Read the model definition and answer for the solid it produces. Units are mm, in the model's axes. Face numbers are marked on the shaded views. A direction names the side the tool comes from. Coordinates: 2 decimals unless noted, no trailing zeros. Write each loop counter-clockwise with the first axis right and the second up, starting at its lowest first coordinate (ties: lowest second). Pieces come first, ordered by that corner, then holes. Notation, with made-up numbers: (32.5, 28.25) -> (64.5, 28.25) arc R13 ccw to (64.5, 53.25) -> close; hole circle Ø4 at (-7.5, -39.75). An arc over 180 degrees is marked (long way). One line per item, written item: value. Start each with the question number.
from build123d import *

# Parameters (mm, degrees)
SKETCH1_W           = 82
SKETCH1_H           = 30
SKETCH1_R           = 2
BOSS_EXTRUDE1_DEPTH = 3
BOSS_EXTRUDE2_DEPTH = 42.5
SKETCH4_R           = 12
SKETCH4_R_2         = 1.65
CUT_EXTRUDE2_DEPTH  = 99.459382488
SKETCH7_W           = 19.5
SKETCH7_H           = 30
CUT_EXTRUDE4_DEPTH  = 98.109474306
SKETCH8_W           = 8
SKETCH8_H           = 5
BOSS_EXTRUDE3_DEPTH = 42.5
SKETCH8_3_R         = 1.755
CUT_EXTRUDE5_DEPTH  = 82.317279836
SKETCH9_W           = 4
SKETCH9_H           = 36
CUT_EXTRUDE6_DEPTH  = 80.26380006
SKETCH10_W          = 46.5
SKETCH10_H          = 46.9
SKETCH10_R          = 4.75
BOSS_EXTRUDE4_DEPTH = 3
BOSS_EXTRUDE4_DRAFT = -33
SKETCH12_W          = 8
SKETCH12_H          = 5
BOSS_EXTRUDE6_DEPTH = 3
CUT_EXTRUDE7_DEPTH  = 3
CUT_EXTRUDE8_DEPTH  = 0.25


with BuildPart() as part:
    # Sketch1 → Boss-Extrude1 (new body)
    with BuildSketch(Plane(origin=(0, 0, 0), x_dir=(1, 0, 0), z_dir=(0, 1, 0))):
        with Locations((41, 15)):
            Rectangle(SKETCH1_W, SKETCH1_H)
        with Locations(Location((78, 23.86, 0), (0, 0, 270))):
            Circle(SKETCH1_R, mode=Mode.SUBTRACT)
        with Locations(Location((78, 5, 0), (0, 0, 270))):
            Circle(SKETCH1_R, mode=Mode.SUBTRACT)
    extrude(amount=BOSS_EXTRUDE1_DEPTH)

    # Sketch2 → Boss-Extrude2 (add)
    with BuildSketch(Plane(origin=(0, 3, 0), x_dir=(1, 0, 0), z_dir=(0, 1, 0))):
        Polygon((52.5, 2.5), (10, 2.5), (10, 30), (8, 30), (8, 0), (54.5, 0), (54.5, 30), (52.5, 30), align=None)
    extrude(amount=BOSS_EXTRUDE2_DEPTH)

    # Sketch4 → Cut-Extrude2 (cut, through all)
    with BuildSketch(Plane.XY):
        with Locations((31.25, 24.25)):
            Circle(SKETCH4_R)
        with Locations((16.25, 9.25)):
            Circle(SKETCH4_R_2)
        with Locations((16.25, 39.25)):
            Circle(SKETCH4_R_2)
        with Locations((46.25, 39.25)):
            Circle(SKETCH4_R_2)
        with Locations((46.25, 9.25)):
            Circle(SKETCH4_R_2)
    extrude(amount=-CUT_EXTRUDE2_DEPTH, mode=Mode.SUBTRACT)

    # Sketch7 → Cut-Extrude4 (cut, through all)
    with BuildSketch(Plane(origin=(0, 3, 0), x_dir=(1, 0, 0), z_dir=(0, 1, 0))):
        with Locations((72.25, 15)):
            Rectangle(SKETCH7_W, SKETCH7_H)
    extrude(amount=-CUT_EXTRUDE4_DEPTH, mode=Mode.SUBTRACT)

    # Sketch8 → Boss-Extrude3 (add)
    with BuildSketch(Plane(origin=(0, 3, 0), x_dir=(1, 0, 0), z_dir=(0, 1, 0))):
        with Locations((4, 15)):
            Rectangle(SKETCH8_W, SKETCH8_H)
        with Locations((58.5, 15)):
            Rectangle(SKETCH8_W, SKETCH8_H)
    extrude(amount=BOSS_EXTRUDE3_DEPTH)

    # Sketch8<3> → Cut-Extrude5 (cut, through all)
    with BuildSketch(Plane(origin=(0, 3, 0), x_dir=(1, 0, 0), z_dir=(0, 1, 0))):
        with Locations(Location((4, 24, 0), (0, 0, 270))):
            Circle(SKETCH8_3_R)
        with Locations(Location((4, 6, 0), (0, 0, 90))):
            Circle(SKETCH8_3_R)
        with Locations(Location((58.5, 6, 0), (0, 0, 270))):
            Circle(SKETCH8_3_R)
        with Locations(Location((58.5, 24, 0), (0, 0, 90))):
            Circle(SKETCH8_3_R)
    extrude(amount=-CUT_EXTRUDE5_DEPTH, mode=Mode.SUBTRACT)

    # Sketch9 → Cut-Extrude6 (cut, through all)
    with BuildSketch(Plane(origin=(0, 0, -17.5), x_dir=(-1, 0, 0), z_dir=(0, 0, -1))):
        with Locations((-58.5, 24.25)):
            Rectangle(SKETCH9_W, SKETCH9_H)
        with Locations((-4, 24.25)):
            Rectangle(SKETCH9_W, SKETCH9_H)
    extrude(amount=-CUT_EXTRUDE6_DEPTH, mode=Mode.SUBTRACT)


with BuildPart() as boss_extrude4_tool:
    # Sketch10 → Boss-Extrude4 (with draft: the straight prism first)
    with BuildSketch(Plane(origin=(0, 45.5, 0), x_dir=(1, 0, 0), z_dir=(0, 1, 0))):
        with Locations((31.25, 23.45)):
            Rectangle(SKETCH10_W, SKETCH10_H)
        with Locations((16.25, 7.5)):
            Circle(SKETCH10_R, mode=Mode.SUBTRACT)
        with Locations((46.25, 7.5)):
            Circle(SKETCH10_R, mode=Mode.SUBTRACT)
        with Locations((46.25, 39.4)):
            Circle(SKETCH10_R, mode=Mode.SUBTRACT)
        with Locations((16.25, 39.4)):
            Circle(SKETCH10_R, mode=Mode.SUBTRACT)
    extrude(amount=BOSS_EXTRUDE4_DEPTH)
    # Boss-Extrude4: the draft: its side faces are tilted about the plane it starts from
    boss_extrude4_sides = [boss_extrude4_tool.faces().sort_by_distance(p)[0] for p in [
        (31.25, 47, 0),
        (54.5, 47, -23.45),
        (31.25, 47, -46.9),
        (8, 47, -23.45),
        (11.5, 47, -7.5),
        (41.5, 47, -7.5),
        (41.5, 47, -39.4),
        (11.5, 47, -39.4),
    ]]
    draft(boss_extrude4_sides, Plane(origin=(0, 45.5, 0), x_dir=(1, 0, 0), z_dir=(0, 1, 0)), BOSS_EXTRUDE4_DRAFT)


with BuildPart() as part_1:
    add(part.part)

    # Boss-Extrude4: add boss_extrude4_tool
    add(boss_extrude4_tool.part)

    # Sketch12 → Boss-Extrude6 (add)
    with BuildSketch(Plane(origin=(0, 45.5, 0), x_dir=(1, 0, 0), z_dir=(0, 1, 0))):
        with Locations((4, 15)):
            Rectangle(SKETCH12_W, SKETCH12_H)
        with Locations((58.5, 15)):
            Rectangle(SKETCH12_W, SKETCH12_H)
    extrude(amount=BOSS_EXTRUDE6_DEPTH)

    # Sketch13 → Cut-Extrude7 (cut)
    with BuildSketch(Plane(origin=(0, 48.5, 0), x_dir=(1, 0, 0), z_dir=(0, 1, 0))):
        Polygon((56.44822278, 17.5), (54.5, 17.5), (54.5, 30), (54.5, 46.9), (8, 46.9), (8, 30), (8, 17.5), (6.05177722, 17.5), (6.05177722, 48.84822278), (56.44822278, 48.84822278), align=None)
        Polygon((54.5, 12.5), (56.44822278, 12.5), (56.44822278, -1.94822278), (6.05177722, -1.94822278), (6.05177722, 12.5), (8, 12.5), (8, 0), (54.5, 0), align=None)
    extrude(amount=-CUT_EXTRUDE7_DEPTH, mode=Mode.SUBTRACT)

    # Sketch15 → Cut-Extrude8 (cut)
    with BuildSketch(Plane.XZ.offset(-45.5)):
        Polygon((10, -2.5), (10, -30), (8, -30), (8, -46.9), (54.5, -46.9), (54.5, -30), (52.5, -30), (52.5, -2.5), align=None)
    extrude(amount=-CUT_EXTRUDE8_DEPTH, mode=Mode.SUBTRACT)


solid = part_1.part
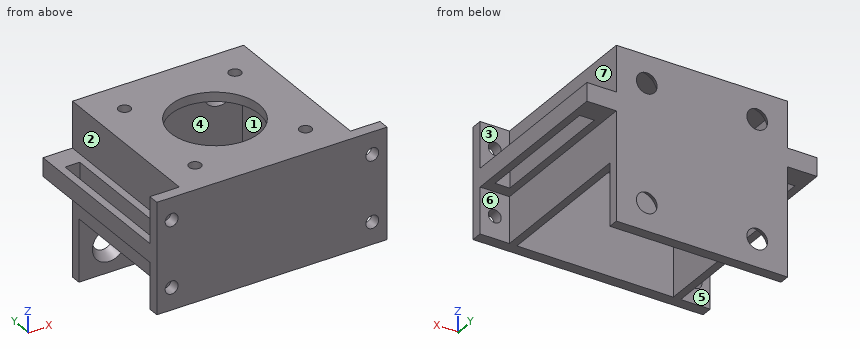
1. Find the intervals of material crossed by probe 1 along X at (y, z) = (1.5, -6) (3 decimals); probe 2 along Y at (x, z) = (46.25, -1); probe 3 along X at (y, z) = (8, -7), in increasing order. Write a range as from..to.
2. A tool of negligible diameter and unlimited length cuts with its end or side. For the marked faces 5, 6 and 7, from which of +Z, -Z, +X, -X, +Y, -Y can it reach the whole face along a straight path? Write none if from no direction.
3. A cutting plane is placed at B-B on z = -14. Give the vertices of the cut face in (x, y), then the cut area to 3 significant figures.
4. A cutting plane is placed at A-A on x = 31.25. Give the vertices of the cut face in (y, z), then the cut area to 3 significant figures.
5. Given pin 1 (9 mm diameter, centred on x = 59.5, z = -4.5, fed in from +Y); pin 2 (1.5 mm diameter, centred on x = 26.5, y = 13.5, fed in from -Z); pin 3 (6 mm diameter, centred on y = 15.5, z = -5.5, fed in from +X), each flat-ended and moving along its own axis, determine where each tip first touches the part or whether it passes through.
6. For a pull along Y with two mould halves and no side action, classify the marked faces 1, 2, 3 and 4 as +Y half, -Y half, draft (parallel to the pull), parting line (faces both ways), or undercut.
7. A cutting plane is placed at D-D on x = 58.5. Give the vertices of the cut face in (y, z) (3 decimals).
8. A cutting plane is placed at C-C on y = 39.25. Count the separate pieces of the cut face and the enclosed holes in it, then the cut area to 3 significant figures.
Derived:
1. probe 1: x = 0..2.245, 5.755..56.745, 60.255..62.5
1. probe 2: y = 0..7.6, 10.9..37.6, 40.9..48.5
1. probe 3: x = 8..10, 52.5..54.5
2. face 5: -Z, -X, +Y
2. face 6: -Z, +X, +Y
2. face 7: +Z, +X, +Y
3. outline: (0, 0) -> (62.5, 0) -> (62.5, 48.5) -> (0, 48.5) -> close; hole (2, 6.25) -> (6, 6.25) -> (6, 42.25) -> (2, 42.25) -> close; hole (10, 3) -> (52.5, 3) -> (52.5, 45.75) -> (10, 45.75) -> close; hole (56.5, 6.25) -> (60.5, 6.25) -> (60.5, 42.25) -> (56.5, 42.25) -> close
3. area: 926 mm2
4. outline: (0, -30) -> (3, -30) -> (3, -2.5) -> (12.25, -2.5) -> (12.25, 0) -> (0, 0) -> close; (36.25, -2.5) -> (45.75, -2.5) -> (45.75, -46.9) -> (48.5, -46.9) -> (48.5, 0) -> (36.25, 0) -> close
4. area: 266 mm2
5. pin 1: stops at y = 3
5. pin 2: stops at z = -2.5
5. pin 3: stops at x = 54.5
6. face 1: undercut
6. face 2: draft
6. face 3: +Y half
6. face 4: undercut
7. outline: (0, -30) -> (3, -30) -> (3, -25.755) -> (0, -25.755) -> close; (0, -22.245) -> (3, -22.245) -> (3, -17.5) -> (6.25, -17.5) -> (6.25, -12.5) -> (3, -12.5) -> (3, -7.755) -> (0, -7.755) -> close; (0, -4.245) -> (3, -4.245) -> (3, 0) -> (0, 0) -> close; (42.25, -17.5) -> (48.5, -17.5) -> (48.5, -12.5) -> (42.25, -12.5) -> close
8. separate pieces: 5
8. enclosed holes: 0
8. area: 250 mm2
